Geometry: final body of the model. Coordinates: model frame, mm. Face numbers are marked on the shaded views. A direction names the side the tool comes from. Coordinates: 2 decimals unless noted, no trailing zeros. Order: outer loops, then holes, each group sorted by start corner. A loop starts at its lowest first (then second) coordinate and runs counter-clockwise, first axis right, second up. Notation, with made-up numbers: M 68.5,-33 L 110.5,-33 A26 cw 110.5,0 Z; hole C 58.25,-6.75 d5. An arc over 180 degrees is marked long. One line per question, with ' | ' between items.
from build123d import *

# Parameters (mm, degrees)
SKETCH_1_W           = 42
SKETCH_1_H           = 14
SKETCH_1_R           = 3
EXTRUDE_1_DEPTH      = 6
SKETCH_2_W           = 20
SKETCH_2_H           = 14
EXTRUDE_2_DEPTH      = 31.5
CUT_EXTRUDE_1_DEPTH  = 37.5
SKETCH_5_R           = 3.5
CUT_EXTRUDE_2_DEPTH  = 2
SKETCH_6_R           = 3.5
SKETCH_6_R_2         = 3
CUT_EXTRUDE_3_DEPTH  = 1
EXTRUDE_3_DEPTH      = 1
EXTRUDE_3_DEPTH_BACK = 15
SKETCH_7_R           = 1.5
SKETCH_8_R           = 1.8
SKETCH_8_R_2         = 1.5
CUT_EXTRUDE_4_DEPTH  = 0.5
CHAMFER_1_SIZE       = 0.5
CHAMFER_2_SIZE       = 0.5
CHAMFER_3_SIZE       = 0.5
CHAMFER_4_SIZE       = 0.5


with BuildPart() as part:
    # 草图1 → 凸台-拉伸1 (new body)
    with BuildSketch(Plane(origin=(0, 0, 0), x_dir=(1, 0, 0), z_dir=(0, 1, 0))):
        with Locations((21, 7)):
            Rectangle(SKETCH_1_W, SKETCH_1_H)
        with Locations(Location((5, 7, 0), (0, 0, 270))):
            Circle(SKETCH_1_R, mode=Mode.SUBTRACT)
        with Locations(Location((37, 7, 0), (0, 0, 270))):
            Circle(SKETCH_1_R, mode=Mode.SUBTRACT)
    extrude(amount=EXTRUDE_1_DEPTH)

    # 草图2 → 凸台-拉伸2 (add)
    with BuildSketch(Plane(origin=(0, 6, 0), x_dir=(1, 0, 0), z_dir=(0, 1, 0))):
        with Locations((21, 7)):
            Rectangle(SKETCH_2_W, SKETCH_2_H)
    extrude(amount=EXTRUDE_2_DEPTH)

    # 草图3 → 切除-拉伸1 (cut)
    with BuildSketch(Plane.XY):
        with BuildLine():
            Line((21.5, 29.480740698), (21.5, 37.5))
            Line((21.5, 37.5), (20.5, 37.5))
            Line((20.5, 37.5), (20.5, 29.480740698))
            ThreePointArc((20.5, 29.480740698), (21, 16.5), (21.5, 29.480740698))
        make_face()
    extrude(amount=-CUT_EXTRUDE_1_DEPTH, mode=Mode.SUBTRACT)

    # 草图5 → 切除-拉伸2 (cut)
    with BuildSketch(Plane(origin=(31, 0, 0), x_dir=(0, 0, -1), z_dir=(1, 0, 0))):
        with Locations((7, 32.5)):
            Circle(SKETCH_5_R)
    extrude(amount=-CUT_EXTRUDE_2_DEPTH, mode=Mode.SUBTRACT)

    # 草图6 → 切除-拉伸3 (cut)
    # profile 1 of 2: a face of its own
    with BuildSketch(Plane(origin=(29, 0, 0), x_dir=(0, 0, -1), z_dir=(1, 0, 0))):
        with Locations((7, 32.5)):
            Circle(SKETCH_6_R)
        with Locations((7, 32.5)):
            Circle(SKETCH_6_R_2, mode=Mode.SUBTRACT)
    # profile 2 of 2: a face of its own
    with BuildSketch(Plane(origin=(29, 0, 0), x_dir=(0, 0, -1), z_dir=(1, 0, 0))):
        Polygon((5.401923789, 31.577350269), (5.401923789, 33.422649731), (7, 34.345299462), (8.598076211, 33.422649731), (8.598076211, 31.577350269), (7, 30.654700538), align=None)
    extrude(amount=-CUT_EXTRUDE_3_DEPTH, mode=Mode.SUBTRACT)

    # 草图7 → 凸台-拉伸3 (add, two sides: drawn at the far end of the back side and taken through both)
    with BuildSketch(Plane.ZY.offset(-11).offset(-EXTRUDE_3_DEPTH_BACK)):
        with Locations((-7, 32.5)):
            Circle(SKETCH_7_R)
    extrude(amount=EXTRUDE_3_DEPTH + EXTRUDE_3_DEPTH_BACK)

    # 草图8 → 切除-拉伸4 (cut)
    with BuildSketch(Plane.ZY.offset(-11)):
        with Locations((-7, 32.5)):
            Circle(SKETCH_8_R)
        with Locations((-7, 32.5)):
            Circle(SKETCH_8_R_2, mode=Mode.SUBTRACT)
    extrude(amount=-CUT_EXTRUDE_4_DEPTH, mode=Mode.SUBTRACT)

    # 倒角1
    chamfer_1_edges = [part.edges().sort_by_distance(p)[0] for p in [
        (11, 32.5, -8.8),
    ]]
    chamfer(chamfer_1_edges, length=CHAMFER_1_SIZE - 0.0001)  # a hair under: the kernel refuses the full size

    # 倒角2
    chamfer_2_edges = [part.edges().sort_by_distance(p)[0] for p in [
        (31, 32.5, -3.5),
    ]]
    chamfer(chamfer_2_edges, length=CHAMFER_2_SIZE)

    # 倒角3
    chamfer_3_edges = [part.edges().sort_by_distance(p)[0] for p in [
        (29, 31.116025404, -7.799038106),
        (29, 32.5, -8.598076211),
        (29, 33.883974596, -7.799038106),
        (29, 33.883974596, -6.200961894),
        (29, 32.5, -5.401923789),
        (29, 31.116025404, -6.200961894),
        (28, 33.883974596, -6.200961894),
        (28, 33.883974596, -7.799038106),
        (28, 32.5, -8.598076211),
        (28, 31.116025404, -7.799038106),
        (28, 31.116025404, -6.200961894),
        (28, 32.5, -5.401923789),
    ]]
    chamfer(chamfer_3_edges, length=CHAMFER_3_SIZE - 0.0001)  # a hair under: the kernel refuses the full size

    # 倒角4
    chamfer_4_edges = [part.edges().sort_by_distance(p)[0] for p in [
        (21, 16.5, 0),
        (21, 16.5, -14),
        (0, 0, -7),
        (0, 6, -7),
        (11, 37.5, -7),
        (31, 37.5, -7),
        (42, 6, -7),
        (15.75, 37.5, 0),
        (11, 21.75, 0),
        (5.5, 6, 0),
        (0, 3, 0),
        (21, 0, 0),
        (26.25, 37.5, 0),
        (31, 21.75, 0),
        (36.5, 6, 0),
        (42, 3, 0),
        (42, 0, -7),
        (26.25, 37.5, -14),
        (31, 21.75, -14),
        (36.5, 6, -14),
        (42, 3, -14),
        (21, 0, -14),
        (0, 3, -14),
        (5.5, 6, -14),
        (11, 21.75, -14),
        (15.75, 37.5, -14),
        (37, 0, -10),
        (37, 6, -10),
        (5, 0, -10),
        (5, 6, -10),
    ]]
    chamfer(chamfer_4_edges, length=CHAMFER_4_SIZE)


solid = part.part
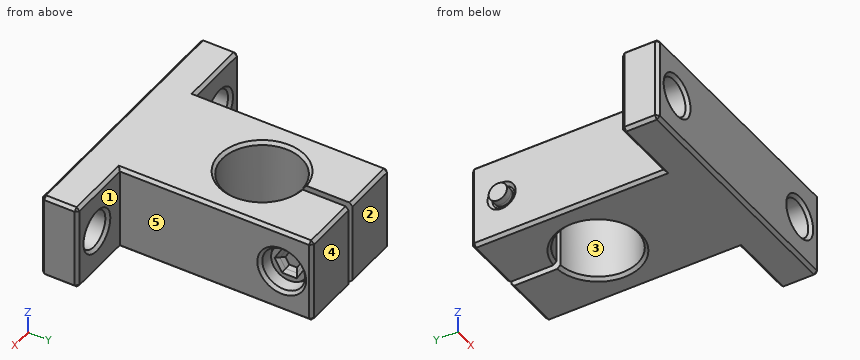
1. Draft query along Y for the marked faces 3, 4 and 5. Return one class per face: pulls with the +Y half, pulls with the -Y half, needs draft (parallel to the pull), parting line crosses it, or undercut.
Response values:
face 3: undercut | face 4: pulls with the +Y half | face 5: needs draft
2. Material intervals for line 1 (X direction, y = 3, z = -7); line 2 (X direction, y = 23, z = -8); line 3 (X direction, y = 7.5, z = -12.75), sorted ascending. Write a range as [from, to].
Response values:
line 1: x = [0, 2], [8, 34], [40, 42] | line 2: x = [11, 14.5], [27.5, 31] | line 3: x = [11, 31]
3. Pin query (flat end, axial travel): P1, Ø4, axis at y = 32.5, z = -7, coming from the +X side; P2, Ø3.5, axis at y = 33.5, z = -6.5, coming from the +X side; P3, Ø5, axis at x = 36.5, z = -10, coming from the +Y side. Return the tip coordinate at first contact, or that it passes through.
Response values:
P1: stops at x = 28.9 | P2: stops at x = 29 | P3: stops at y = 6
4. Section A-A, the plane y = 4. Output: boundary loops of the cut face in (x, z).
Response values:
outline: M 0,-13.5 L 0.5,-14 L 41.5,-14 L 42,-13.5 L 42,-0.5 L 41.5,0 L 0.5,0 L 0,-0.5 Z; hole C 5,-7 d6; hole C 37,-7 d6
5. Access query for the marked faces 1 and 2. Directions: +Z, -Z, +X, -X, +Y, -Y. A direction counts if a zero-diameter tool reaches every point of the face in a straight line with its end or side. Return the directions, or none.
Response values:
face 1: +Z, -Z, +X, +Y | face 2: +Z, -Z, +X, -X, +Y
6. Section B-B, the plane x = 21. Output: boundary loops of the cut face in (y, z).
Response values:
outline: M 0,-13.5 L 0.5,-14 L 16,-14 L 16.5,-13.5 L 16.5,-0.5 L 16,0 L 0.5,0 L 0,-0.5 Z; C 32.5,-7 d3
7. Section C-C, the plane z = -12. Output: boundary loops of the cut face in (x, y).
Response values:
outline: M 0,0.5 L 0.5,0 L 41.5,0 L 42,0.5 L 42,5.5 L 41.5,6 L 31,6 L 31,37 L 30.5,37.5 L 21.5,37.5 L 21.5,29.48 A6.5 cw long 20.5,29.48 L 20.5,37.5 L 11.5,37.5 L 11,37 L 11,6 L 0.5,6 L 0,5.5 Z
8. Section D-D, the plane y = 23. Output: boundary loops of the cut face in (x, z).
Response values:
outline: M 11,-13.5 L 11.5,-14 L 14,-14 L 14.5,-13.5 L 14.5,-0.5 L 14,0 L 11.5,0 L 11,-0.5 Z; M 27.5,-13.5 L 28,-14 L 30.5,-14 L 31,-13.5 L 31,-0.5 L 30.5,0 L 28,0 L 27.5,-0.5 Z
